```python
from build123d import *

# Parameters (mm, degrees)
SKETCH1_R           = 8
BOSS_EXTRUDE1_DEPTH = 7.4
SKETCH2_R           = 5.95
BOSS_EXTRUDE2_DEPTH = 7
SKETCH3_R           = 8
BOSS_EXTRUDE3_DEPTH = 1
SKETCH4_R           = 2.35
CUT_EXTRUDE1_DEPTH  = 21


with BuildPart() as part:
    # Sketch1 → Boss-Extrude1 (new body)
    with BuildSketch(Plane(origin=(0, 0, 0), x_dir=(1, 0, 0), z_dir=(0, 1, 0))):
        Circle(SKETCH1_R)
    extrude(amount=BOSS_EXTRUDE1_DEPTH)

    # Sketch2 → Boss-Extrude2 (add)
    with BuildSketch(Plane(origin=(0, 7.4, 0), x_dir=(1, 0, 0), z_dir=(0, 1, 0))):
        Circle(SKETCH2_R)
    extrude(amount=BOSS_EXTRUDE2_DEPTH)

    # Sketch3 → Boss-Extrude3 (add)
    with BuildSketch(Plane(origin=(0, 14.4, 0), x_dir=(1, 0, 0), z_dir=(0, 1, 0))):
        Circle(SKETCH3_R)
    extrude(amount=BOSS_EXTRUDE3_DEPTH)

    # Sketch4 → Cut-Extrude1 (cut)
    with BuildSketch(Plane.XZ):
        Circle(SKETCH4_R)
    extrude(amount=-CUT_EXTRUDE1_DEPTH, mode=Mode.SUBTRACT)


solid = part.part
```
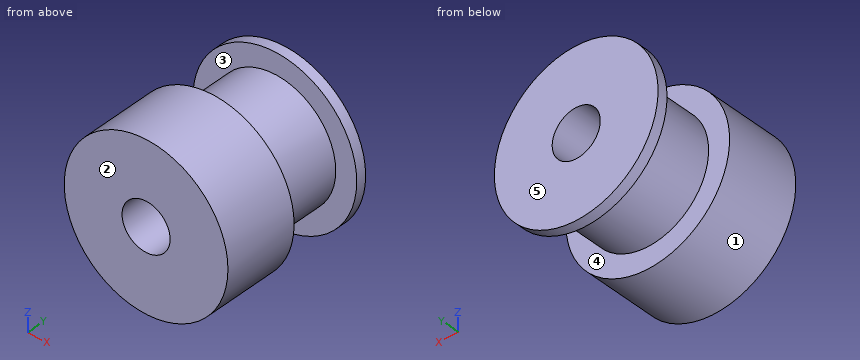
For this review, take the finished solid that the model builds, in its own axes (mm). Face numbers are marked on the shaded views. A direction names the side the tool comes from. Coordinates: 2 decimals unless noted, no trailing zeros. Loops run counter-clockwise (first coordinate to the right, second up) from the corner with the lowest first, then second, coordinate; pieces in that order, holes last.
1. Add section B-B, the plane x = 0. Give the boundary of the cut face in (y, z).
2. Insertion check: P1, Ø6, axis at y = 3, z = -3, coming from the -X side; P2, Ø3, axis at y = 5.5, z = 2, coming from the +X side; P3, Ø2, axis at x = 4, y = 3.5, coming from the +Z side; P4, Ø8, axis at y = 11, z = -3.5, coming from the +X side. Each pin has a flat end and moves straight along its axis. Give the tip position at first contact, or say it passes through.
3. For line 1 (Y direction, x = 4, z = 6); line 2 (Z direction, x = 0, y = 10); line 3 (Z direction, x = 0, y = 7.25), list the stretches that pass through material, from the lowest coordinate up.
4. Add section D-D, the plane z = 4.75. Give the boundary of the cut face in (x, y).
5. Add section A-A, the plane z = 0. Give the boundary of the cut face in (x, y).
6. For the marked faces 4 and 5, list the 3-axis set-ups (+Z, -Z, +X, -X, +Y, -Y) from which the entire face can be reached by the end or side of a thin tool; tool diameter is ignored.
7. Add section C-C, the plane y = 8.5. Give the boundary of the cut face in (x, z).
8. Mouldability with a two-part tool opening along Y and no side actions: class the marked faces 1, 2 and 3 as +Y half, -Y half, draft (parallel to the pull), parting line (faces both ways), or undercut.
Result:
1. outline: (0, -8) - (7.4, -8) - (7.4, -5.95) - (14.4, -5.95) - (14.4, -8) - (15.4, -8) - (15.4, -2.35) - (0, -2.35) - close; (0, 2.35) - (15.4, 2.35) - (15.4, 8) - (14.4, 8) - (14.4, 5.95) - (7.4, 5.95) - (7.4, 8) - (0, 8) - close
2. P1: stops at x = -8
2. P2: stops at x = 7.98
2. P3: stops at z = 7.42
2. P4: stops at x = 7.88
3. line 1: y = 0 to 7.4, 14.4 to 15.4
3. line 2: z = -5.95 to -2.35, 2.35 to 5.95
3. line 3: z = -8 to -2.35, 2.35 to 8
4. outline: (-6.44, 0) - (6.44, 0) - (6.44, 7.4) - (3.58, 7.4) - (3.58, 14.4) - (6.44, 14.4) - (6.44, 15.4) - (-6.44, 15.4) - (-6.44, 14.4) - (-3.58, 14.4) - (-3.58, 7.4) - (-6.44, 7.4) - close
5. outline: (-8, 0) - (-2.35, 0) - (-2.35, 15.4) - (-8, 15.4) - (-8, 14.4) - (-5.95, 14.4) - (-5.95, 7.4) - (-8, 7.4) - close; (2.35, 0) - (8, 0) - (8, 7.4) - (5.95, 7.4) - (5.95, 14.4) - (8, 14.4) - (8, 15.4) - (2.35, 15.4) - close
6. face 4: none
6. face 5: +Z, -Z, +X, -X, +Y
7. outline: circle Ø11.9 at (0, 0); hole circle Ø4.7 at (0, 0)
8. face 1: draft
8. face 2: -Y half
8. face 3: undercut
